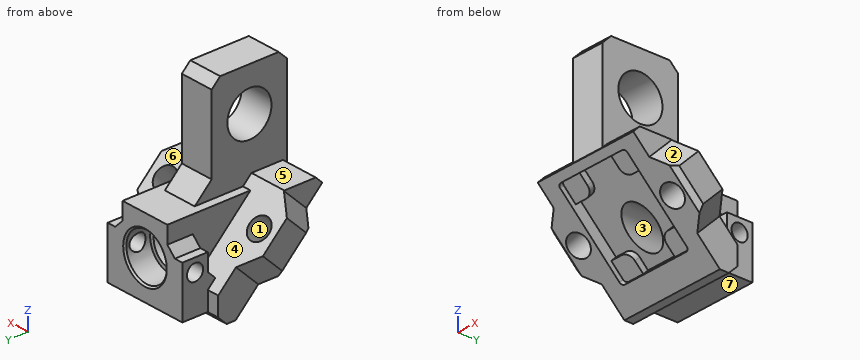
```python
from build123d import *

# Parameters (mm, degrees)
SKETCH2_W                = 4.5
SKETCH2_H                = 5.27595021
BOSS_EXTRUDE1_DEPTH      = 1.5
BOSS_EXTRUDE2_DEPTH      = 3.2
CUT_EXTRUDE1_DEPTH       = 7.4
SKETCH5_R                = 1.3
BOSS_EXTRUDE3_DEPTH      = 1
BOSS_EXTRUDE4_DEPTH      = 1.86
SKETCH7_R                = 0.65
CUT_EXTRUDE2_DEPTH       = 10.564291115
SKETCH8_W                = 4.5
SKETCH8_H                = 5.34
CUT_EXTRUDE3_DEPTH       = 0.7
FILLET1_R                = 0.2
SKETCH9_W                = 1.19
SKETCH9_H                = 1.19
BOSS_EXTRUDE5_DEPTH      = 0.4
FILLET2_R                = 0.5
BOSS_EXTRUDE6_DEPTH      = 2.5
SKETCH10_R               = 0.925
CUT_EXTRUDE4_DEPTH       = 1
CUT_EXTRUDE4_DEPTH_BACK  = 8.63704148
M1_2X0_25_TAPPED_HOLE1_D = 0.95
CHAMFER1_SIZE            = 0.5
SKETCH14_R               = 1.36
CUT_EXTRUDE5_DEPTH       = 1.5
CHAMFER2_SIZE            = 0.2
CHAMFER3_SIZE            = 0.1
CHAMFER4_SIZE            = 0.25


with BuildPart() as part:
    # Sketch2 → Boss-Extrude1 (new body, symmetric)
    with BuildSketch(Plane(origin=(0, 0, 0), x_dir=(0, 0, -1), z_dir=(1, 0, 0))):
        with Locations((0, 2.637975105)):
            Rectangle(SKETCH2_W, SKETCH2_H)
    extrude(amount=BOSS_EXTRUDE1_DEPTH, both=True)

    # Sketch3 → Boss-Extrude2 (add, symmetric)
    with BuildSketch(Plane(origin=(0, 0, 0), x_dir=(0, 0, -1), z_dir=(1, 0, 0))):
        Polygon((0, 0), (2.75, 2.75), (2.75, 3.27595021), (2.25, 3.77595021), (1.145512984, 3.77595021), (-2.75, -0.119562774), (-2.75, -1.972182541), (-2.36109127, -2.36109127), align=None)
    extrude(amount=BOSS_EXTRUDE2_DEPTH, both=True)

    # Sketch4 → Cut-Extrude1 (cut, through all)
    with BuildSketch(Plane(origin=(3.2, 0, 0), x_dir=(0, 0, -1), z_dir=(1, 0, 0))):
        Polygon((2.25, 2.25), (0, 0), (2.25, 0), align=None)
    extrude(amount=-CUT_EXTRUDE1_DEPTH, mode=Mode.SUBTRACT)

    # Sketch5 → Boss-Extrude3 (add, symmetric)
    with BuildSketch(Plane(origin=(0, 0, 0), x_dir=(0, 0, -1), z_dir=(1, 0, 0))):
        Polygon((-2.497182541, -2.225), (-7.75, -2.225), (-8.25, -1.725), (-8.25, 1.725), (-7.75, 2.225), (-3.25, 2.225), (-2.25, 3.225), (-2.25, 0.380437226), (-2.75, -0.119562774), (-2.75, -1.972182541), align=None)
        with Locations((-5.75, 0)):
            Circle(SKETCH5_R, mode=Mode.SUBTRACT)
    extrude(amount=BOSS_EXTRUDE3_DEPTH, both=True)

    # Sketch6 → Boss-Extrude4 (add)
    with BuildSketch(Plane(origin=(0, 0, 0), x_dir=(1, 0, 0), z_dir=(0, -0.707106781, -0.707106781))):
        Polygon((-3.2, 2), (-4.2, 1), (-4.2, -1), (-3.2, -2), align=None)
        Polygon((3.2, -2), (3.2, 2), (4.2, 1), (4.2, -1), align=None)
    extrude(amount=-BOSS_EXTRUDE4_DEPTH)

    # Sketch7 → Cut-Extrude2 (cut, through all)
    with BuildSketch(Plane(origin=(0, 0, 0), x_dir=(1, 0, 0), z_dir=(0, -0.707106781, -0.707106781))):
        with Locations((-3.15, 0)):
            Circle(SKETCH7_R)
        with Locations((3.15, 0)):
            Circle(SKETCH7_R)
    extrude(amount=-CUT_EXTRUDE2_DEPTH, mode=Mode.SUBTRACT)

    # Sketch8 → Cut-Extrude3 (cut)
    with BuildSketch(Plane(origin=(0, 0, 0), x_dir=(1, 0, 0), z_dir=(0, -0.707106781, -0.707106781))):
        with Locations((0, 0.17)):
            Rectangle(SKETCH8_W, SKETCH8_H)
    extrude(amount=-CUT_EXTRUDE3_DEPTH, mode=Mode.SUBTRACT)

    # Fillet1
    fillet1_edges = [part.edges().sort_by_distance(p)[0] for p in [
        (-2.25, 2.015254326, -1.52027958),
        (-2.25, -1.760695885, 2.255670632),
        (2.25, -1.760695885, 2.255670632),
        (2.25, 2.015254326, -1.52027958),
    ]]
    fillet(fillet1_edges, radius=FILLET1_R)

    # Sketch9 → Boss-Extrude5 (add)
    with BuildSketch(Plane(origin=(0, 0.494974747, 0.494974747), x_dir=(1, 0, 0), z_dir=(0, -0.707106781, -0.707106781))):
        with Locations((-1.655, 2.245)):
            Rectangle(SKETCH9_W, SKETCH9_H)
        with Locations((1.655, 2.245)):
            Rectangle(SKETCH9_W, SKETCH9_H)
        with Locations((1.655, -1.905)):
            Rectangle(SKETCH9_W, SKETCH9_H)
        with Locations((-1.655, -1.905)):
            Rectangle(SKETCH9_W, SKETCH9_H)
    extrude(amount=BOSS_EXTRUDE5_DEPTH)

    # Fillet2
    fillet2_edges = [part.edges().sort_by_distance(p)[0] for p in [
        (-1.06, -0.813172798, 1.52027958),
        (1.06, -0.813172798, 1.52027958),
        (1.06, 1.279863274, -0.572756493),
        (-1.06, 1.279863274, -0.572756493),
    ]]
    fillet(fillet2_edges, radius=FILLET2_R)

    # Sketch11 → Boss-Extrude6 (add, symmetric)
    with BuildSketch(Plane(origin=(0, 0, 0), x_dir=(0, 0, -1), z_dir=(1, 0, 0))):
        Polygon((2.25, 5.27595021), (-0.75, 5.27595021), (-0.75, 3.77595021), (0.25, 3.77595021), (0.697756492, 3.328193718), (1.145512984, 3.77595021), (2.25, 3.77595021), align=None)
    extrude(amount=BOSS_EXTRUDE6_DEPTH, both=True)

    # Sketch10 → Cut-Extrude4 (cut, two sides)
    with BuildSketch(Plane(origin=(0, 5.27595021, 0), x_dir=(1, 0, 0), z_dir=(0, 1, 0))) as cut_extrude4_sk:
        Circle(SKETCH10_R)
    extrude(amount=CUT_EXTRUDE4_DEPTH, mode=Mode.SUBTRACT)
    extrude(cut_extrude4_sk.sketch, amount=-CUT_EXTRUDE4_DEPTH_BACK, mode=Mode.SUBTRACT)

    # M1.2x0.25 Tapped Hole1 (through all)
    with Locations(Plane(origin=(2.5, 0, 0), x_dir=(0, 0, -1), z_dir=(1, 0, 0))):
        with Locations((0, 4.52595021)):
            Hole(M1_2X0_25_TAPPED_HOLE1_D / 2)

    # Chamfer1
    chamfer1_edges = [part.edges().sort_by_distance(p)[0] for p in [
        (1.5, 4.52595021, 0.75),
        (-1.5, 4.52595021, 0.75),
    ]]
    chamfer(chamfer1_edges, length=CHAMFER1_SIZE)

    # Sketch14 → Cut-Extrude5 (cut)
    with BuildSketch(Plane(origin=(0, 5.27595021, 0), x_dir=(1, 0, 0), z_dir=(0, 1, 0))):
        Circle(SKETCH14_R)
    extrude(amount=-CUT_EXTRUDE5_DEPTH, mode=Mode.SUBTRACT)

    # Chamfer2
    chamfer2_edges = [part.edges().sort_by_distance(p)[0] for p in [
        (-0.925, 3.77595021, 0),
    ]]
    chamfer(chamfer2_edges, length=CHAMFER2_SIZE)

    # Chamfer3
    chamfer3_edges = [part.edges().sort_by_distance(p)[0] for p in [
        (-1.36, 5.27595021, 0),
    ]]
    chamfer(chamfer3_edges, length=CHAMFER3_SIZE)

    # Chamfer4
    chamfer4_edges = [part.edges().sort_by_distance(p)[0] for p in [
        (4.2, 0, 0),
        (-4.2, 0, 0),
    ]]
    chamfer(chamfer4_edges, length=CHAMFER4_SIZE)


solid = part.part
```
Geometry check sheet. Reference: the model listing, model coordinates, mm. Face numbers are marked on the shaded views. A direction names the side the tool comes from. Round coordinates to 2 decimals unless told otherwise and drop trailing zeros. Order: outer loops, then holes, each group sorted by start corner. A loop starts at its lowest first (then second) coordinate and runs counter-clockwise, first axis right, second up. Notation, with made-up numbers: M -20,8 L 35,8 A36 cw 35,43 Z; hole C 15,24.25 d3. An arc over 180 degrees is marked long. Write item = value, one per line.
Q1. Scan lines: line 1 (Z direction, x = 0, y = 4.75); line 2 (X direction, y = 1.25, z = 1); line 3 (Y direction, x = -1.9, z = 0). Record each from-to range of solid material in increasing order.
Answer block:
line_1 = -2.25 to -1.36, 1.36 to 2.25
line_2 = -4.2 to -3.78, -2.52 to 2.52, 3.78 to 4.2
line_3 = 0.99 to 2.63, 3.78 to 4.05, 5 to 5.28
Q2. Section check C-C (x = 3). Enter the section's corners in (y, z).
Answer block:
outline = M -2.36,2.36 L -0.45,0.45 L 0.87,1.76 L -0.12,2.75 L -1.97,2.75 Z; M 0.45,-0.45 L 2.75,-2.75 L 3.28,-2.75 L 3.78,-2.25 L 3.78,-1.15 L 1.76,0.87 Z
Q3. Section check B-B (z = 5.75). Enter the section's corners in (x, y) (3 decimals), plus the area to 3 significant figures.
Answer block:
outline = M -1,-2.225 L 1,-2.225 L 1,-1.3 L -1,-1.3 Z; M -1,1.3 L 1,1.3 L 1,2.225 L -1,2.225 Z
area = 3.70 mm^2
Q4. Set-up check for the marked faces 5, 6 and 7: record each of +Z, -Z, +X, -X, +Y, -Y from which the full face is reachable in a straight line by a thin tool's end or side.
Answer block:
face_5 = +Z, -X, +Y, -Y
face_6 = +Z, +X
face_7 = -Z, +X, -X, +Y
Q5. Release check for a two-part mould opening along Y. For the marked faces 1, 2, 3 and 4 record: released by +Y, released by -Y, zero draft, split by the parting line, or undercut.
Answer block:
face_1 = undercut
face_2 = released by -Y
face_3 = zero draft
face_4 = undercut
Q6. Depth check by flat-ended pin: pin 1 Ø2 at (x, y) = (3.5, 0) entering from +Z; pin 2 Ø1.2 at (y, z) = (2.5, -1) entering from -X; pin 3 Ø0.8 at (x, y) = (0.5, 4.5) entering from -Z; pin 4 Ø1.1 at (y, z) = (-1, 0) entering from -X. Enter the tip coordinate at first touch or a pass-through.
Answer block:
pin_1 = 2.75
pin_2 = -3.33
pin_3 = -2.25
pin_4 = through
Q7. Section check A-A (x = 0). Give the number of separate pieces and of enclosed holes in the cut face, plus the area to 3 significant figures.
Answer block:
separate_pieces = 2
enclosed_holes = 1
area = 32.9 mm^2
